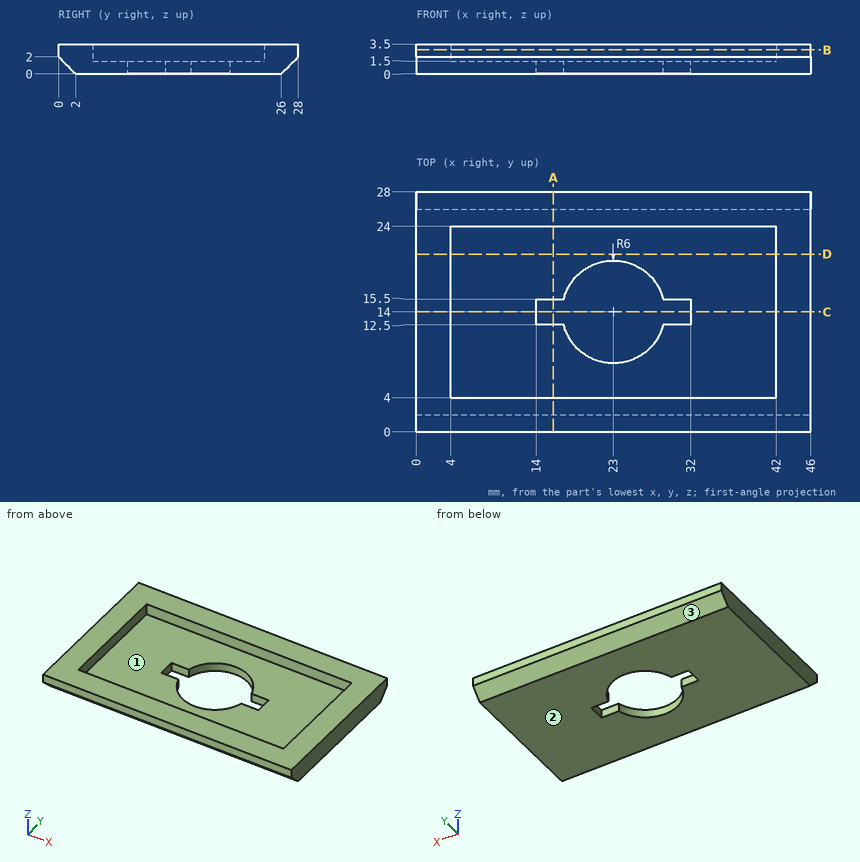
Drawing for the job (mm, zero at the part's lowest x, y, z). Round coordinates to 2 decimals unless told otherwise and drop trailing zeros. Write each loop counter-clockwise with the first axis right and the second up, starting at its lowest first coordinate (ties: lowest second). Pieces come first, ordered by that corner, then holes. Notation, with made-up numbers: (21.5, 69.5) - (38.5, 69.5) arc R30 ccw to (38.5, 101.5) - close; hole circle Ø5 at (-35.5, 47.5). An arc over 180 degrees is marked (long way). Return JSON: item names as keys, results as strings. Group by question number.
Item 1: Band-saw the part on D-D on y = 20.75. List the corners of the cut face in (x, z).
Item 2: Probe probe 1 along X at (y, z) = (14, 2.8); probe 2 along Y at (x, z) = (34, 3); probe 3 along Z at (x, y) = (10, 4.5). List the from-to ranges inside material, lowest first.
Item 3: Band-saw the part on A-A on x = 16. List the corners of the cut face in (y, z).
Item 4: Flat gauge pins, fed straight in: pin 1 Ø0.8 at (x, z) = (16.5, 0.5) entering from +Y; pin 2 Ø0.8 at (x, z) = (16.5, 0.5) entering from -Y; pin 3 Ø1.6 at (x, z) = (30.5, 0.5) entering from +Y. Where does each tip first touch, or does it go through?
Item 5: Band-saw the part on C-C on y = 14. List the corners of the cut face in (x, z).
Item 6: Band-saw the part on B-B on z = 2.8. List the corners of the cut face in (x, y).
Item 7: Mould opens along Y. For the marked faces 1, 2 and 3 say: +Y half, -Y half, draft (parallel to the pull), parting line (faces both ways), or undercut.
Resolved:
{
 "1": {"outline": "(0, 0) - (46, 0) - (46, 3.5) - (42, 3.5) - (42, 1.5) - (4, 1.5) - (4, 3.5) - (0, 3.5) - close"},
 "2": {"probe 1": "x = 0 to 4, 42 to 46", "probe 2": "y = 0 to 4, 24 to 28", "probe 3": "z = 0 to 1.5"},
 "3": {"outline": "(0, 2) - (2, 0) - (12.5, 0) - (12.5, 1.5) - (4, 1.5) - (4, 3.5) - (0, 3.5) - close; (15.5, 0) - (26, 0) - (28, 2) - (28, 3.5) - (24, 3.5) - (24, 1.5) - (15.5, 1.5) - close"},
 "4": {"pin 1": "stops at y = 26.9", "pin 2": "stops at y = 1.1", "pin 3": "stops at y = 27.3"},
 "5": {"outline": "(0, 0) - (14, 0) - (14, 1.5) - (4, 1.5) - (4, 3.5) - (0, 3.5) - close; (32, 0) - (46, 0) - (46, 3.5) - (42, 3.5) - (42, 1.5) - (32, 1.5) - close"},
 "6": {"outline": "(0, 0) - (46, 0) - (46, 28) - (0, 28) - close; hole (4, 4) - (42, 4) - (42, 24) - (4, 24) - close"},
 "7": {"face 1": "undercut", "face 2": "draft", "face 3": "+Y half"}
}
